Can you work these out from the model? Positions are in its coordinate system, mm. Face numbers are marked on the shaded views. A direction names the side the tool comes from. Give positions to 0.01 mm unless a question says otherwise; leave off trailing zeros. Loops run counter-clockwise (first coordinate to the right, second up) from the corner with the lowest first, then second, coordinate; pieces in that order, holes last. Notation, with made-up numbers: M 73.5,70 L 111.5,70 A10 ccw 111.5,78 Z; hole C 48.5,-30.75 d5. An arc over 180 degrees is marked long. Put each result on its own line as item: value. Start each with the question number.
1) Imagine slicing it at D-D (z = 4.25). Write out the boundary of the cut face in (x, y).
2) For P1, Ø3, axis at x = 7.38, z = 2.5, coming from the -Y side; P2, Ø1.5, axis at x = 8, z = 3.5, coming from the +Y side; P3, Ø2.5, axis at x = 6.5, z = 2.5, coming from the -Y side, each with a flat end and sliding along its axis, tell me the tip position at first contact or that it passes through.
3) If we mould it in two halves opening along Y, with no side actions, what happens to the marked faces 3, 4 and 5? For each: +Y half, -Y half, draft (parallel to the pull), parting line (faces both ways), or undercut.
4) For the marked faces 1 and 2, which set-ups out of +Z, -Z, +X, -X, +Y, -Y let a thin tool reach every point of the face, with its end or its side?
5) Please list where these lines run through material, in increasing order: line 1 along Y through (x, z) = (8.75, 1.3); line 2 along Y through (x, z) = (0, 3.2); line 3 along X through (y, z) = (1.25, 2). Write a range as from..to.
6) Imagine slicing it at C-C (y = 2). State how many separate pieces and enclosed holes the cut face has, then the cut area to 3 significant figures.
7) Imagine slicing it at B-B (z = 2). Write out the boundary of the cut face in (x, y), then the cut area to 3 significant figures.
8) Imagine slicing it at A-A (x = 6). Write out the boundary of the cut face in (y, z).
from build123d import *

# Parameters (mm, degrees)
BOSS_EXTRUDE1_DEPTH     = 5
FILLET3_R               = 1
FILLET4_R               = 1
CUT_EXTRUDE1_DEPTH      = 13.854889966
CUT_EXTRUDE1_DEPTH_BACK = 13.854889966
SKETCH2_R               = 1


with BuildPart() as part:
    # Sketch1 → Boss-Extrude1 (new body)
    with BuildSketch(Plane(origin=(0, 0, 0), x_dir=(0, 1, 0), z_dir=(0, 0, 1))):
        with BuildLine():
            Line((-0.977144637, -2.88923664), (-0.977144637, -6.118433409))
            Line((-0.977144637, -6.118433409), (-0.977144637, -9.381714775))
            Line((-0.977144637, -9.381714775), (-3.05, -9.381714775))
            Line((-3.05, -9.381714775), (-3.05, -5.455272679))
            ThreePointArc((-3.05, -5.455272679), (-0.035341977, 6.249900075), (3.1115, -5.420430587))
            Line((3.1115, -5.420430587), (3.1115, -9.381714775))
            Line((3.1115, -9.381714775), (1.022855363, -9.381714775))
            Line((1.022855363, -9.381714775), (1.022855363, -6.104337812))
            Line((1.022855363, -6.104337812), (1.022855363, -2.873372044))
            ThreePointArc((1.022855363, -2.873372044), (-0.024192746, 3.049904049), (-0.977144637, -2.88923664))
        make_face()
    extrude(amount=BOSS_EXTRUDE1_DEPTH)

    # Fillet3
    fillet3_edges = [part.edges().sort_by_distance(p)[0] for p in [
        (-6.249900075, -0.035341977, 5),
    ]]
    fillet(fillet3_edges, radius=FILLET3_R)

    # Fillet4
    fillet4_edges = [part.edges().sort_by_distance(p)[0] for p in [
        (-6.249900075, -0.035341977, 0),
    ]]
    fillet(fillet4_edges, radius=FILLET4_R)

    # Sketch2 → Cut-Extrude1 (cut, two sides: drawn at the far end of the back side and taken through both)
    with BuildSketch(Plane(origin=(0, -0.977144637, 0), x_dir=(-1, 0, 0), z_dir=(0, 1, 0)).offset(-CUT_EXTRUDE1_DEPTH_BACK)):
        with Locations(Location((-7.381714775, 2.5, 0), (0, 0, 180))):
            Circle(SKETCH2_R)
    extrude(amount=CUT_EXTRUDE1_DEPTH + CUT_EXTRUDE1_DEPTH_BACK, mode=Mode.SUBTRACT)


solid = part.part
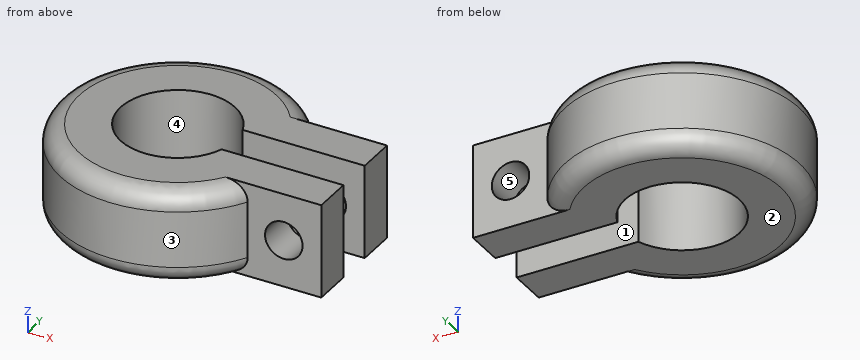
Recorded:
1. outline: M 2.87,1.02 L 9.38,1.02 L 9.38,3.11 L 5.38,3.11 A6.22 ccw long 5.42,-3.05 L 9.38,-3.05 L 9.38,-0.98 L 2.89,-0.98 A3.05 cw long Z
2. P1: y = -3.05
2. P2: y = 3.11
2. P3: y = -3.39
3. face 3: parting line
3. face 4: undercut
3. face 5: draft
4. face 1: +Z, -Z, +X
4. face 2: -Z, +X, -X, +Y, -Y
5. line 1: -3.05..-0.98, 1.02..3.11
5. line 2: -6.25..-3.05, 3.05..6.25
5. line 3: -6.12..-2.78, 2.78..6.52, 8.25..9.38
6. separate pieces: 2
6. enclosed holes: 1
6. area: 49.9 mm²
7. outline: M 2.87,1.02 L 6.52,1.02 L 6.52,3.11 L 5.42,3.11 A6.25 ccw long 5.46,-3.05 L 6.52,-3.05 L 6.52,-0.98 L 2.89,-0.98 A3.05 cw long Z; M 8.25,-3.05 L 9.38,-3.05 L 9.38,-0.98 L 8.25,-0.98 Z; M 8.25,1.02 L 9.38,1.02 L 9.38,3.11 L 8.25,3.11 Z
7. area: 94.4 mm²
8. outline: M -3.05,0 L -0.98,0 L -0.98,5 L -3.05,5 Z; M 1.02,0 L 3.11,0 L 3.11,5 L 1.02,5 Z
